Geometry check sheet. Reference: the model listing, model coordinates, mm. A direction names the side the tool comes from. Give positions to 0.01 mm unless a question says otherwise; leave off trailing zeros. Order: outer loops, then holes, each group sorted by start corner. A loop starts at its lowest first (then second) coordinate and runs counter-clockwise, first axis right, second up. Notation, with made-up numbers: M 6.5,78.25 L 13.5,78.25 A7 ccw 13.5,88.25 Z; hole C 31,46 d3. An arc over 180 degrees is marked long. Answer as CSV lines item,"result". Start each with the question number.
```python
from build123d import *

# Parameters (mm, degrees)
SKETCH1_R           = 11.049
SKETCH1_R_2         = 4.05
BOSS_EXTRUDE1_DEPTH = 3.937
SKETCH2_R           = 9.4615
SKETCH2_R_2         = 5.6375
CUT_EXTRUDE1_DEPTH  = 0.381


with BuildPart() as part:
    # Sketch1 → Boss-Extrude1 (new body, symmetric)
    with BuildSketch(Plane.XY):
        Circle(SKETCH1_R)
        Circle(SKETCH1_R_2, mode=Mode.SUBTRACT)
    extrude(amount=BOSS_EXTRUDE1_DEPTH, both=True)

    # Sketch2 → Cut-Extrude1 (cut)
    with BuildSketch(Plane.XY.offset(3.937)):
        Circle(SKETCH2_R)
        Circle(SKETCH2_R_2, mode=Mode.SUBTRACT)
    cut_extrude1 = extrude(amount=-CUT_EXTRUDE1_DEPTH, mode=Mode.SUBTRACT)

    # Mirror1: Cut-Extrude1 across plane
    add(cut_extrude1.mirror(Plane.XY), mode=Mode.SUBTRACT)


solid = part.part
```
Item 1: Section check C-C on z = 1.5. Record the boundary of the cut face in (x, y), then the cut area to 3 significant figures.
Item 2: Section check D-D on y = 6.5. Record the boundary of the cut face in (x, z), then the cut area to 3 significant figures.
Item 3: Depth check by flat-ended pin: pin 1 Ø3 at (y, z) = (-4, -2) entering from -X; pin 2 Ø3 at (y, z) = (5, 0.5) entering from -X; pin 3 Ø1.5 at (x, z) = (-2.5, 3) entering from -Y. Enter the tip coordinate at first touch or a pass-through.
Item 4: Draft check along X on faces 4 (the face through (3.031, 4.754, 3.749)), 5 (the face through (-4.96, 8.24, -3.937)), 6 (the face through (-1.438, 10.955, 0.055)). Enter one of: pulls with the +X half, pulls with the -X half, needs draft (parallel to the pull), parting line crosses it, or undercut.
Item 5: Access from +Z, -Z, +X, -X, +Y, -Y to the whole of each face (thin tool, end or side, straight path). Record for faces 1 (the face through (3.031, 4.754, -3.749)), 2 (the face through (4.1, -4.1, 3.556)), 3 (the face through (2, -4, -3.937)).
Item 6: Section check A-A on y = 0. Record the boundary of the cut face in (x, z).
Item 7: Scan lines: line 1 along Y through (x, z) = (0, 3.85); line 2 along Y through (x, z) = (0, 0); line 3 along Z through (x, y) = (-6, -2.75). Record each from-to range of solid material in increasing order.
Numbers:
1,outline,"C 0,0 d22.1; hole C 0,0 d8.1"
1,area,"332 mm2"
2,outline,"M -8.93,-3.94 L -6.88,-3.94 L -6.88,-3.56 L 6.88,-3.56 L 6.88,-3.94 L 8.93,-3.94 L 8.93,3.94 L 6.88,3.94 L 6.88,3.56 L -6.88,3.56 L -6.88,3.94 L -8.93,3.94 Z"
2,area,"130 mm2"
3,pin 1,"x = -10.76"
3,pin 2,"x = -10.48"
3,pin 3,"y = -10.91"
4,face 4,"undercut"
4,face 5,"needs draft"
4,face 6,"parting line crosses it"
5,face 1,"-Z"
5,face 2,"+Z"
5,face 3,"-Z, +X, -X, +Y, -Y"
6,outline,"M -11.05,-3.94 L -9.46,-3.94 L -9.46,-3.56 L -5.64,-3.56 L -5.64,-3.94 L -4.05,-3.94 L -4.05,3.94 L -5.64,3.94 L -5.64,3.56 L -9.46,3.56 L -9.46,3.94 L -11.05,3.94 Z; M 4.05,-3.94 L 5.64,-3.94 L 5.64,-3.56 L 9.46,-3.56 L 9.46,-3.94 L 11.05,-3.94 L 11.05,3.94 L 9.46,3.94 L 9.46,3.56 L 5.64,3.56 L 5.64,3.94 L 4.05,3.94 Z"
7,line 1,"-11.05 to -9.46, -5.64 to -4.05, 4.05 to 5.64, 9.46 to 11.05"
7,line 2,"-11.05 to -4.05, 4.05 to 11.05"
7,line 3,"-3.56 to 3.56"
